Can you work these out from the model? Positions are in its coordinate system, mm. Face numbers are marked on the shaded views. Give positions to 0.01 mm unless a question says otherwise; leave off trailing zeros. Order: outer loops, then holes, each group sorted by start corner. A loop starts at its lowest first (then second) coordinate and runs counter-clockwise, first axis right, second up. Notation, with made-up numbers: (30, -23.5) -> (85, -23.5) arc R24 ccw to (85, 3.5) -> close; hole circle Ø8 at (-32.75, -4.5). An arc over 180 degrees is marked (long way). Answer as a JSON object with one key per item and string values.
```python
from build123d import *

# Parameters (mm, degrees)
PAD014_DEPTH                       = 3.9
SKETCH022_R                        = 2.4
POCKET007_DEPTH                    = 7.8
LINEARPATTERN007_COUNT             = 6
LINEARPATTERN007_PITCH             = 8
SKETCH023_R                        = 3.1
POCKET008_DEPTH                    = 0.8
SKETCH023_LINEARPATTERN008_2_R     = 3.1
POCKET008_LINEARPATTERN008_2_DEPTH = 0.8
SKETCH023_LINEARPATTERN008_3_R     = 3.1
POCKET008_LINEARPATTERN008_3_DEPTH = 0.8
SKETCH023_LINEARPATTERN008_4_R     = 3.1
POCKET008_LINEARPATTERN008_4_DEPTH = 0.8
SKETCH023_LINEARPATTERN008_5_R     = 3.1
POCKET008_LINEARPATTERN008_5_DEPTH = 0.8
SKETCH023_LINEARPATTERN008_6_R     = 3.1
POCKET008_LINEARPATTERN008_6_DEPTH = 0.8
BODY005_PLACEMENT_ANGLE            = 90


with BuildPart() as part:
    # Sketch021 → Pad014 (new body, symmetric)
    with BuildSketch(Plane.XY):
        with BuildLine():
            Line((-20, 3.9), (20, 3.9))
            ThreePointArc((20, -3.9), (23.9, 0), (20, 3.9))
            Line((20, -3.9), (-20, -3.9))
            ThreePointArc((-20, 3.9), (-23.9, 0), (-20, -3.9))
        make_face()
    extrude(amount=PAD014_DEPTH, both=True)

    # Sketch022 (on Face6 of Pad014) → Pocket007 (cut)
    with BuildSketch(Plane.XY.offset(3.9)):
        with Locations((20, 0)):
            Circle(SKETCH022_R)
    pocket007 = extrude(amount=-POCKET007_DEPTH, mode=Mode.SUBTRACT)

    # LinearPattern007: Pocket007 ×6
    with Locations(*[(-i * LINEARPATTERN007_PITCH, 0, 0) for i in range(1, LINEARPATTERN007_COUNT)]):
        add(pocket007, mode=Mode.SUBTRACT)

    # Sketch023 (on Face5 of LinearPattern007) → Pocket008 (cut)
    with BuildSketch(Plane.XY.offset(3.9)):
        with Locations((20, 0)):
            Circle(SKETCH023_R)
    pocket008 = extrude(amount=-POCKET008_DEPTH, mode=Mode.SUBTRACT)

    # Sketch023 LinearPattern008 2 → Pocket008 LinearPattern008 2 (cut)
    with BuildSketch(Plane(origin=(-8, 0, 3.9), x_dir=(1, 0, 0), z_dir=(0, 0, 1))):
        with Locations((20, 0)):
            Circle(SKETCH023_LINEARPATTERN008_2_R)
    pocket008_linearpattern008_2 = extrude(amount=-POCKET008_LINEARPATTERN008_2_DEPTH, mode=Mode.SUBTRACT)

    # Sketch023 LinearPattern008 3 → Pocket008 LinearPattern008 3 (cut)
    with BuildSketch(Plane(origin=(-16, 0, 3.9), x_dir=(1, 0, 0), z_dir=(0, 0, 1))):
        with Locations((20, 0)):
            Circle(SKETCH023_LINEARPATTERN008_3_R)
    pocket008_linearpattern008_3 = extrude(amount=-POCKET008_LINEARPATTERN008_3_DEPTH, mode=Mode.SUBTRACT)

    # Sketch023 LinearPattern008 4 → Pocket008 LinearPattern008 4 (cut)
    with BuildSketch(Plane(origin=(-24, 0, 3.9), x_dir=(1, 0, 0), z_dir=(0, 0, 1))):
        with Locations((20, 0)):
            Circle(SKETCH023_LINEARPATTERN008_4_R)
    pocket008_linearpattern008_4 = extrude(amount=-POCKET008_LINEARPATTERN008_4_DEPTH, mode=Mode.SUBTRACT)

    # Sketch023 LinearPattern008 5 → Pocket008 LinearPattern008 5 (cut)
    with BuildSketch(Plane(origin=(-32, 0, 3.9), x_dir=(1, 0, 0), z_dir=(0, 0, 1))):
        with Locations((20, 0)):
            Circle(SKETCH023_LINEARPATTERN008_5_R)
    pocket008_linearpattern008_5 = extrude(amount=-POCKET008_LINEARPATTERN008_5_DEPTH, mode=Mode.SUBTRACT)

    # Sketch023 LinearPattern008 6 → Pocket008 LinearPattern008 6 (cut)
    with BuildSketch(Plane(origin=(-40, 0, 3.9), x_dir=(1, 0, 0), z_dir=(0, 0, 1))):
        with Locations((20, 0)):
            Circle(SKETCH023_LINEARPATTERN008_6_R)
    pocket008_linearpattern008_6 = extrude(amount=-POCKET008_LINEARPATTERN008_6_DEPTH, mode=Mode.SUBTRACT)

    # Mirrored003: Pocket008, Pocket008 LinearPattern008 2, Pocket008 LinearPattern008 3, Pocket008 LinearPattern008 4, Pocket008 LinearPattern008 5, Pocket008 LinearPattern008 6 across XY
    add(pocket008.mirror(Plane.XY), mode=Mode.SUBTRACT)
    add(pocket008_linearpattern008_2.mirror(Plane.XY), mode=Mode.SUBTRACT)
    add(pocket008_linearpattern008_3.mirror(Plane.XY), mode=Mode.SUBTRACT)
    add(pocket008_linearpattern008_4.mirror(Plane.XY), mode=Mode.SUBTRACT)
    add(pocket008_linearpattern008_5.mirror(Plane.XY), mode=Mode.SUBTRACT)
    add(pocket008_linearpattern008_6.mirror(Plane.XY), mode=Mode.SUBTRACT)


with BuildPart() as part_1:
    # Body005 placement: moved
    add(part.part.moved(Location((0, 20, 20))).rotate(Axis((0, 20, 20), (0, 0, 1)), BODY005_PLACEMENT_ANGLE))


solid = part_1.part
```
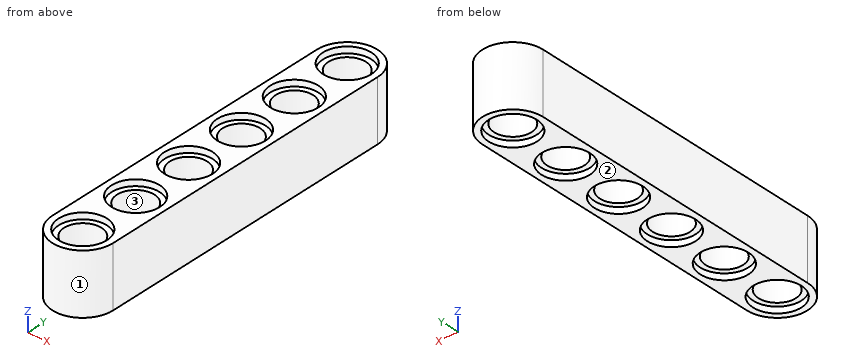
1. If we mould it in two halves opening along X, with no side actions, what happens to the marked faces 1, 2 and 3? For each: +X half, -X half, draft (parallel to the pull), parting line (faces both ways), or undercut.
Worked answers:
{"face 1": "parting line", "face 2": "draft", "face 3": "undercut"}
2. Please list where these lines run through material, in increasing order: L1, parallel to X at y = 24, z = 16.6; L2, parallel to X at y = 0, z = 20.5; L3, parallel to Z at x = 2, y = 34.
Worked answers:
{"L1": "-3.9 to -3.1, 3.1 to 3.9", "L2": "-3.9 to -2.4, 2.4 to 3.9", "L3": "16.9 to 23.1"}
3. If we section it at D-D on y = 22: Please give me the cut outline in (x, z).
Worked answers:
{"outline": "(-3.9, 16.1) -> (-2.37, 16.1) -> (-2.37, 16.9) -> (-1.33, 16.9) -> (-1.33, 23.1) -> (-2.37, 23.1) -> (-2.37, 23.9) -> (-3.9, 23.9) -> close; (1.33, 16.9) -> (2.37, 16.9) -> (2.37, 16.1) -> (3.9, 16.1) -> (3.9, 23.9) -> (2.37, 23.9) -> (2.37, 23.1) -> (1.33, 23.1) -> close"}
4. If we section it at A-A on y = 32: Please give me the cut outline in (x, z).
Worked answers:
{"outline": "(-3.9, 16.1) -> (-3.1, 16.1) -> (-3.1, 16.9) -> (-2.4, 16.9) -> (-2.4, 23.1) -> (-3.1, 23.1) -> (-3.1, 23.9) -> (-3.9, 23.9) -> close; (2.4, 16.9) -> (3.1, 16.9) -> (3.1, 16.1) -> (3.9, 16.1) -> (3.9, 23.9) -> (3.1, 23.9) -> (3.1, 23.1) -> (2.4, 23.1) -> close"}
5. If we section it at B-B on z = 23.5: Please give me the cut outline in (x, y), then the cut area to 3 significant figures.
Worked answers:
{"outline": "(-3.9, 0) arc R3.9 ccw to (3.9, 0) -> (3.9, 40) arc R3.9 ccw to (-3.9, 40) -> close; hole circle Ø6.2 at (0, 0); hole circle Ø6.2 at (0, 8); hole circle Ø6.2 at (0, 16); hole circle Ø6.2 at (0, 24); hole circle Ø6.2 at (0, 32); hole circle Ø6.2 at (0, 40)", "area": "179 mm²"}
6. If we section it at C-C on x = -1.25: Count the separate pieces of the cut face and the enclosed holes in it, then the cut area to 3 significant figures.
Worked answers:
{"separate pieces": "7", "enclosed holes": "0", "area": "163 mm²"}
7. Will this pin go through, and if not, where does the flat tip stop? pin 1 Ø3 at (x, y) = (0.5, 41) entering from +Z.
Worked answers:
{"pin 1": "z = 23.1"}
